Read the model definition and answer for the solid it produces. Units are mm, in the model's axes. Coordinates: 2 decimals unless noted, no trailing zeros. Loops run counter-clockwise (first coordinate to the right, second up) from the corner with the lowest first, then second, coordinate; pieces in that order, holes last. Notation, with made-up numbers: M -11,-37.5 L 35,-37.5 A13 cw 35,-22.5 Z; hole C 39.5,8 d7. An arc over 180 degrees is marked long. Put each result on its own line as item: value.
from build123d import *

# Parameters (mm, degrees)
BOSS_EXTRU_1_DEPTH      = 3
ESQUISSE2_R             = 1.5
ENL_V_MAT_EXTRU_2_DEPTH = 3
ESQUISSE3_R             = 6
ESQUISSE3_R_2           = 1.5
ENL_V_MAT_EXTRU_3_DEPTH = 10
ESQUISSE4_W             = 100
ESQUISSE4_H             = 11.457187309
ENL_V_MAT_EXTRU_4_DEPTH = 10


with BuildPart() as part:
    # Esquisse1 → Boss.-Extru.1 (new body)
    with BuildSketch(Plane.XY):
        Polygon((-50, -75), (50, -75), (50, -65), (60, -65), (60, 75), (-60, 75), (-60, -65), (-50, -65), align=None)
        with BuildLine():
            ThreePointArc((-41.5, 22), (-43, 20.5), (-44.5, 22))
            Line((-44.5, 22), (-44.5, 37))
            ThreePointArc((-44.5, 37), (-43, 38.5), (-41.5, 37))
            Line((-41.5, 37), (-41.5, 22))
        make_face(mode=Mode.SUBTRACT)
        with BuildLine():
            Line((-10.5, 37), (-10.5, 22))
            ThreePointArc((-10.5, 22), (-12, 20.5), (-13.5, 22))
            Line((-13.5, 22), (-13.5, 37))
            ThreePointArc((-13.5, 37), (-12, 38.5), (-10.5, 37))
        make_face(mode=Mode.SUBTRACT)
        with BuildLine():
            ThreePointArc((-41.5, 53), (-43, 51.5), (-44.5, 53))
            Line((-44.5, 53), (-44.5, 68))
            ThreePointArc((-44.5, 68), (-43, 69.5), (-41.5, 68))
            Line((-41.5, 68), (-41.5, 53))
        make_face(mode=Mode.SUBTRACT)
        with BuildLine():
            ThreePointArc((-16.25, 37.5), (-27.5, 26.25), (-38.75, 37.5))
            Line((-38.75, 37.5), (-38.75, 52.5))
            ThreePointArc((-38.75, 52.5), (-27.5, 63.75), (-16.25, 52.5))
            Line((-16.25, 52.5), (-16.25, 37.5))
        make_face(mode=Mode.SUBTRACT)
        with BuildLine():
            Line((-10.5, 68), (-10.5, 53))
            ThreePointArc((-10.5, 53), (-12, 51.5), (-13.5, 53))
            Line((-13.5, 53), (-13.5, 68))
            ThreePointArc((-13.5, 68), (-12, 69.5), (-10.5, 68))
        make_face(mode=Mode.SUBTRACT)
    extrude(amount=BOSS_EXTRU_1_DEPTH)

    # Esquisse2 → Enlèv. mat.-Extru.2 (cut)
    with BuildSketch(Plane.XY.offset(3)):
        with Locations((45, -70)):
            Circle(ESQUISSE2_R)
        with Locations((-55, -60)):
            Circle(ESQUISSE2_R)
        with Locations((-55, 5)):
            Circle(ESQUISSE2_R)
        with Locations((-55, 70)):
            Circle(ESQUISSE2_R)
        with Locations((22.5, -70)):
            Circle(ESQUISSE2_R)
        with Locations((0, -70)):
            Circle(ESQUISSE2_R)
        with Locations((-22.5, -70)):
            Circle(ESQUISSE2_R)
        with Locations((-45, -70)):
            Circle(ESQUISSE2_R)
        with Locations(Location((55, -60, 0), (0, 0, 180))):
            Circle(ESQUISSE2_R)
        with Locations(Location((55, 5, 0), (0, 0, 180))):
            Circle(ESQUISSE2_R)
        with Locations(Location((55, 70, 0), (0, 0, 180))):
            Circle(ESQUISSE2_R)
    extrude(amount=-ENL_V_MAT_EXTRU_2_DEPTH, mode=Mode.SUBTRACT)

    # Esquisse3 → Enlèv. mat.-Extru.3 (cut)
    with BuildSketch(Plane.XY.offset(3)):
        with Locations((0, -40)):
            Circle(ESQUISSE3_R)
        with Locations((-7.5, -32.5)):
            Circle(ESQUISSE3_R_2)
        with Locations((7.5, -32.5)):
            Circle(ESQUISSE3_R_2)
        with Locations((7.5, -47.5)):
            Circle(ESQUISSE3_R_2)
        with Locations((-7.5, -47.5)):
            Circle(ESQUISSE3_R_2)
    extrude(amount=-ENL_V_MAT_EXTRU_3_DEPTH, mode=Mode.SUBTRACT)

    # Esquisse4 → Enlèv. mat.-Extru.4 (cut)
    with BuildSketch(Plane.XY.offset(3)):
        with Locations((0, -70.728593655)):
            Rectangle(ESQUISSE4_W, ESQUISSE4_H)
    extrude(amount=-ENL_V_MAT_EXTRU_4_DEPTH, mode=Mode.SUBTRACT)


solid = part.part
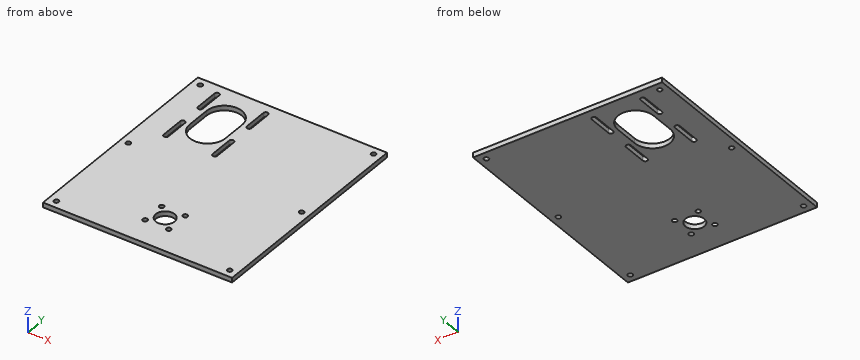
1) Find section B-B, the plane y = -32.5. Write down the section's boundary in (x, z).
Answer list:
outline: M -60,0 L -9,0 L -9,3 L -60,3 Z; M -6,0 L 6,0 L 6,3 L -6,3 Z; M 9,0 L 60,0 L 60,3 L 9,3 Z
2) Given pin 1 Ø2.5 at (x, y) = (55, 70) entering from -Z, flat-ended and moving along its own axis, determine where the tip first touches the part or whether it passes through.
Answer list:
pin 1: passes through
3) Find section A-A, the plane x = -36.5. Write down the section's boundary in (y, z), plus the area to 4 significant figures.
Answer list:
outline: M -65,0 L 30.75,0 L 30.75,3 L -65,3 Z; M 59.25,0 L 75,0 L 75,3 L 59.25,3 Z
area: 334.5 mm^2
4) Find section C-C, the plane x = 7.5. Write down the section's boundary in (y, z).
Answer list:
outline: M -65,0 L -49,0 L -49,3 L -65,3 Z; M -46,0 L -34,0 L -34,3 L -46,3 Z; M -31,0 L 75,0 L 75,3 L -31,3 Z
5) Find section D-D, the plane z = 1.75. Count the separate pieces of the cut face and the enclosed holes in it, plus the area to 3 significant figures.
Answer list:
separate pieces: 1
enclosed holes: 16
area: 15,700 mm^2
6) Straight lines are drawn through the part: line 1 (X direction, y = 70, z = 0.95); line 2 (Y direction, x = -7.5, z = 1); line 3 (Y direction, x = -43, z = 2.15). For each, find the intervals that lie inside material, in ascending order. Write a range as [from, to].
Answer list:
line 1: x = [-60, -56.5], [-53.5, 53.5], [56.5, 60]
line 2: y = [-65, -49], [-46, -34], [-31, 75]
line 3: y = [-65, 20.5], [38.5, 51.5], [69.5, 75]
